Build history of the part. All positions in model axes, mm. A direction names the side the tool comes from. Coordinates: 2 decimals unless noted, no trailing zeros. Loops run counter-clockwise (first coordinate to the right, second up) from the corner with the lowest first, then second, coordinate; pieces in that order, holes last.
(1) Slice it at D-D (z = 4). Give the cut face in (x, y).
(2) Wall check: L1, parallel to Y at x = 7, z = 5.25; L2, parallel to X at y = 6, z = 4.75; L3, parallel to Y at x = 4.75, z = 6. Give the ranges that are in metal, low to high.
(3) Slice it at C-C (x = -1). Give the cut face in (y, z), and give its area (3 significant figures).
(4) Flat gauge pins, fed straight in: P1, Ø1, axis at x = -1, y = 9.5, coming from the -Z side; P2, Ø1.6, axis at x = 5, y = -11, coming from the +Z side; P3, Ø3, axis at x = 1, y = 2, coming from the +Z side. Where does each tip first touch, or does it go through?
(5) Two-plate mould, pull along X, no slides. Class faces 1 (the face through (-0.04, 14.55, 1.57)), 2 (the face through (5, -10, 5)), 3 (the face through (-7.5, 0, 4)): pulls with the +X half, pulls with the -X half, needs draft (parallel to the pull), parting line crosses it, or undercut.
(6) Slice it at A-A (z = 6.25). Give the cut face in (x, y).
(7) Tool access for faces 4 (the face through (-5, 10, 5)), 5 (the face through (-7.07, -10.23, 4.55)), 6 (the face through (4.93, -14.55, 5.27)), 7 (the face through (4.5, 0, 5)): list every direction of +Z, -Z, +X, -X, +Y, -Y with a clear straight run to the whole face (end or side of a thin tool).
(8) Slice it at B-B (y = 11.5). Give the cut face in (x, z), and give its area (3 significant figures).
Solid Edge part; units mm, degrees
sketch "Sketch1" plane through (0, 0, 0) normal (0, -1, 0) x (1, 0, 0)
  line L0 (7.5, 2) -> (4.5, 2)
  line L1 (4.5, 2) -> (4.5, 7)
  line L2 (4.5, 7) -> (7.5, 7)
  line L3 (7.5, 7) -> (7.5, 2)
  line L4 (-4.5, 2) -> (-4.5, 7)
  line L5 (-4.5, 7) -> (-7.5, 7)
  line L6 (-7.5, 7) -> (-7.5, 2)
  line L7 (-7.5, 2) -> (-4.5, 2)
  line L8 (7.5, 2) -> (-7.5, 2)
  line L9 (-7.5, 2) -> (-7.5, 0)
  line L10 (-7.5, 0) -> (7.5, 0)
  line L11 (7.5, 0) -> (7.5, 2)
extrude "Protrusion1" add sketch "Sketch1" along normal mid plane 30
sketch "Sketch2" plane through (0, 0, 0) normal (1, 0, 0) x (0, 1, 0)
  line L0 (-12, 0) -> (-8.5, 0)
  line L1 (-8.5, 0) -> (-8.5, 1.1151)
  line L2 (-8.5, 1.1151) -> (-12, 1.1151)
  line L3 (-12, 1.1151) -> (-12, 0)
  line L4 (8.5, 5) -> (8.5, 9.3332)
  line L5 (8.5, 9.3332) -> (12, 9.3332)
  line L6 (12, 9.3332) -> (12, 5)
  line L7 (12, 5) -> (8.5, 5)
  line L8 (8.5, 1.1151) -> (12, 1.1151)
  line L9 (12, 1.1151) -> (12, 0)
  line L10 (12, 0) -> (8.5, 0)
  line L11 (8.5, 0) -> (8.5, 1.1151)
  line L12 (-8.5, 9.3332) -> (-8.5, 5)
  line L13 (-8.5, 5) -> (-12, 5)
  line L14 (-12, 5) -> (-12, 9.3332)
  line L15 (-12, 9.3332) -> (-8.5, 9.3332)
extrude "Cutout1" cut sketch "Sketch2" against normal up to next and the other way up to next
fillet "Round_1" radius 1.75 1 edges at (-7.5, 10.25, 1.1151)
fillet "Round_1" radius 1.5 13 edges at (-4.5, 0, 2) (4.5, 0, 2) (0, 15, 2) (-4.5, 15, 4.5) (4.5, 15, 4.5) (-4.5, -15, 4.5) (4.5, -15, 4.5) (0, -15, 2) (-7.5, -10.25, 5) (7.5, -10.25, 5) (7.5, 10.25, 5) (-7.5, 10.25, 5) (7.5, 10.25, 1.1151)
Response values:
1. outline: (-7.5, -15) - (-6, -15) arc R1.5 ccw to (-4.5, -13.5) - (-4.5, 13.5) arc R1.5 ccw to (-6, 15) - (-7.5, 15) - (-7.5, 12) - (-7.41, 12) - (-7.41, 8.5) - (-7.5, 8.5) - (-7.5, -8.5) - (-7.41, -8.5) - (-7.41, -12) - (-7.5, -12) - close; (4.5, -13.5) arc R1.5 ccw to (6, -15) - (7.5, -15) - (7.5, -12) - (7.41, -12) - (7.41, -8.5) - (7.5, -8.5) - (7.5, 8.5) - (7.41, 8.5) - (7.41, 12) - (7.5, 12) - (7.5, 15) - (6, 15) arc R1.5 ccw to (4.5, 13.5) - close
2. L1: y = -15 to -12, -8.5 to 8.5, 12 to 15
2. L2: x = -7.5 to -4.5, 4.5 to 7.5
2. L3: y = -14.33 to -12, -8.5 to 8.5, 12 to 14.33
3. outline: (-15, 0) - (-12, 0) - (-12, 1.12) - (-8.5, 1.12) - (-8.5, 0) - (8.5, 0) - (8.5, 1.12) - (12, 1.12) - (12, 0) - (15, 0) - (15, 0.5) arc R1.5 ccw to (13.5, 2) - (-13.5, 2) arc R1.5 ccw to (-15, 0.5) - close
3. area: 51.2 mm2
4. P1: stops at z = 1.12
4. P2: stops at z = 5
4. P3: stops at z = 2
5. face 1: undercut
5. face 2: needs draft
5. face 3: pulls with the -X half
6. outline: (-7.5, -15) - (-6, -15) arc R1.5 ccw to (-4.5, -13.5) - (-4.5, -12) - (-7.5, -12) - close; (-7.5, -8.5) - (-4.5, -8.5) - (-4.5, 8.5) - (-7.5, 8.5) - close; (-7.5, 12) - (-4.5, 12) - (-4.5, 13.5) arc R1.5 ccw to (-6, 15) - (-7.5, 15) - close; (4.5, -13.5) arc R1.5 ccw to (6, -15) - (7.5, -15) - (7.5, -12) - (4.5, -12) - close; (4.5, -8.5) - (7.5, -8.5) - (7.5, 8.5) - (4.5, 8.5) - close; (4.5, 12) - (7.5, 12) - (7.5, 15) - (6, 15) arc R1.5 ccw to (4.5, 13.5) - close
7. face 4: +Z, +X, -X
7. face 5: +Z, -X
7. face 6: +Z, -Y
7. face 7: +Z, +Y, -Y
8. outline: (-7.5, 2.87) arc R1.75 ccw to (-5.75, 1.12) - (6, 1.12) arc R1.5 ccw to (7.5, 2.62) - (7.5, 3.5) arc R1.5 ccw to (6, 5) - (4.5, 5) - (4.5, 3.5) arc R1.5 cw to (3, 2) - (-3, 2) arc R1.5 cw to (-4.5, 3.5) - (-4.5, 5) - (-6, 5) arc R1.5 ccw to (-7.5, 3.5) - close
8. area: 30.1 mm2
